Input: part model. Units: mm. Frame: model coordinates. A direction names the side the tool comes from. Coordinates: 2 decimals unless noted, no trailing zeros. Loops run counter-clockwise (first coordinate to the right, second up) from the corner with the lowest first, then second, coordinate; pieces in that order, holes last. Notation, with made-up numbers: M -26.75,3.25 L 6.25,3.25 A14 ccw 6.25,25.25 Z; hole C -16,-12 d5. An arc over 180 degrees is marked long. Use a Markdown table: item, result. Add a question column.
1. Section A-A on y = -12.5. Output: boundary loops of the cut face in (x, z), then the cut area to 3 significant figures.
2. Section B-B on z = -4.5. Output: boundary loops of the cut face in (x, y).
3. Set-up query: faces 4 (the flat face through (8.792, -96, 11)), 5 (the flat face through (-4, -96, 14.569)), 6 (the flat face through (-8.792, -96, 11)), 7 (the flat face through (-5, -53, 6.9)), 8 (the flat face through (4.3, -195, 6.5)). Return all of +Z, -Z, +X, -X, +Y, -Y with unobstructed straight access to the full face (end or side cutting, diameter ignored); none if empty.
4. Draft query along Y for faces 1 (the flat face through (5, -53, 6.9)), 2 (the flat face through (4, -96, 14.569)), 3 (the flat face through (4.3, 0, 6.5)). Return one class per face: +Y half, -Y half, draft (parallel to the pull), parting line (faces both ways), or undercut.
5. Pin query (flat end, axial travel): pin 1 (9.5 mm diameter, centred on y = -113.5, z = 10, fed in from +X); pin 2 (3 mm diameter, centred on y = -165.5, z = 6, fed in from +X); pin 3 (4 mm diameter, centred on x = 2.5, y = -144.5, fed in from -Z); pin 4 (8 mm diameter, centred on x = 0, y = -89, fed in from +Z). Return the tip coordinate at first contact, or that it passes through.
6. Line query: L1, parallel to Z at x = -0.75, y = -35; L2, parallel to Z at x = -5.5, y = -75; L3, parallel to X at y = -111, z = 0. Output: solid intervals per line, ascending. Write a range as [from, to].
```python
from build123d import *

# Parameters (mm, degrees)
F0_R     = 10
F0_R_2   = 7.5
F1_DEPTH = 195
F2_R     = 7.5
F3_DEPTH = 25
F4_W     = 25.85132
F4_H     = 17
F5_DEPTH = 25
F6_DEPTH = 6.9
F8_DEPTH = 195


with BuildPart() as f1:
    # F0 (on Front) → F1 (new body)
    with BuildSketch(Plane.XZ):
        Circle(F0_R)
        Circle(F0_R_2, mode=Mode.SUBTRACT)
    extrude(amount=F1_DEPTH)

    # F2 (on Top) → F3 (cut)
    with BuildSketch(Plane.XY):
        with Locations((0, -22.5)):
            Circle(F2_R)
    extrude(amount=-F3_DEPTH, mode=Mode.SUBTRACT)

    # F4 (on Top) → F5 (cut)
    with BuildSketch(Plane.XY):
        with Locations((0, -53.5)):
            Rectangle(F4_W, F4_H)
    extrude(amount=-F5_DEPTH, mode=Mode.SUBTRACT)

    # F4 (on Top) → F6 (cut)
    with BuildSketch(Plane.XY):
        with Locations((0, -53.5)):
            Rectangle(F4_W, F4_H)
    extrude(amount=F6_DEPTH, mode=Mode.SUBTRACT)

    # F7 (on Front) → F8 (join)
    with BuildSketch(Plane.XZ):
        with BuildLine():
            ThreePointArc((6.1, 7.924014), (7.611905, 6.485284), (8.79225, 4.764068))
            Line((8.79225, 4.764068), (8.79225, 5.520866))
            Line((8.79225, 5.520866), (8.79225, 16.675162))
            Line((8.79225, 16.675162), (1.726435, 16.675162))
            Line((1.726435, 16.675162), (1.726435, 14.56902))
            Line((1.726435, 14.56902), (6.1, 14.56902))
            Line((6.1, 14.56902), (6.1, 10.11902))
            Line((6.1, 10.11902), (6.1, 7.924014))
        make_face()
        with BuildLine():
            Line((-8.79225, 5.520866), (-8.79225, 4.764068))
            ThreePointArc((-8.79225, 4.764068), (-7.611905, 6.485284), (-6.1, 7.924014))
            Line((-6.1, 7.924014), (-6.1, 10.11902))
            Line((-6.1, 10.11902), (-6.1, 14.56902))
            Line((-6.1, 14.56902), (-1.726435, 14.56902))
            Line((-1.726435, 14.56902), (-1.726435, 16.675162))
            Line((-1.726435, 16.675162), (-8.79225, 16.675162))
            Line((-8.79225, 16.675162), (-8.79225, 5.520866))
        make_face()
        with BuildLine():
            Line((-6.1, 10.11902), (-6.1, 7.924014))
            ThreePointArc((-6.1, 7.924014), (0, 10), (6.1, 7.924014))
            Line((6.1, 7.924014), (6.1, 10.11902))
            Line((6.1, 10.11902), (-6.1, 10.11902))
        make_face()
    extrude(amount=F8_DEPTH)


solid = f1.part
```
Answers below:
| question | item | result |
|---|---|---|
| 1 | outline | M -8.79,4.76 A10 ccw long 8.79,4.76 L 8.79,16.68 L 1.73,16.68 L 1.73,14.57 L 6.1,14.57 L 6.1,10.12 L -6.1,10.12 L -6.1,14.57 L -1.73,14.57 L -1.73,16.68 L -8.79,16.68 Z; hole C 0,0 d15 |
| 1 | area | 220 mm² |
| 2 | outline | M -8.93,-195 L -6,-195 L -6,-62 L -8.93,-62 Z; M -8.93,-45 L -6,-45 L -6,-27 A7.5 cw -6,-18 L -6,0 L -8.93,0 Z; M 6,-195 L 8.93,-195 L 8.93,-62 L 6,-62 Z; M 6,-45 L 8.93,-45 L 8.93,0 L 6,0 L 6,-18 A7.5 cw 6,-27 Z |
| 3 | face 4 | +Z, +X, +Y, -Y |
| 3 | face 5 | +Y, -Y |
| 3 | face 6 | +Z, -X, +Y, -Y |
| 3 | face 7 | -Z |
| 3 | face 8 | +Z, -Z, +X, -X, -Y |
| 4 | face 1 | undercut |
| 4 | face 2 | draft |
| 4 | face 3 | +Y half |
| 5 | pin 1 | stops at x = 8.79 |
| 5 | pin 2 | stops at x = 8.93 |
| 5 | pin 3 | stops at z = -9.99 |
| 5 | pin 4 | stops at z = 16.68 |
| 6 | L1 | z = [-9.97, -7.46], [7.46, 10.12] |
| 6 | L2 | z = [-8.35, -5.1], [5.1, 10.12], [14.57, 16.68] |
| 6 | L3 | x = [-10, -7.5], [7.5, 10] |
